Autodesk Inventor part; units mm, degrees
ref_plane "Arbeitsebene1" through (0, 1.75, 0) normal (0, 1, 0) x (-1, 0, 0)
ref_plane "YZ Plane" through (0, 0, 0) normal (1, 0, 0) x (0, 1, 0)
ref_plane "XY Plane" through (0, 0, 0) normal (0, 0, 1) x (1, 0, 0)
sketch "Skizze1" plane through (0, 0, 0) normal (0, 1, 0) x (-1, 0, 0)
  line L0 (0, 0) -> (1.5, 0)
  line L1 (1.5, 0) -> (1.5, -6.5)
  line L2 (1.5, -6.5) -> (2, -6.5)
  line L3 (2, -6.5) -> (2, -36.5)
  line L4 (0, 0) -> (0, -44)
  line L5 (2, -36.5) -> (1.5, -36.5)
  line L6 (1.5, -36.5) -> (1.5, -42.5)
  arc A0 (0, -44) -> (1.5, -42.5) centre (0, -42.5) ccw
  point P0 (0, -26.7554)
  dimension "d0" = 6.5
  dimension "d1" = 3
  dimension "d2" = 4
  dimension "d5" = 30
  dimension "d6" = 0.5
  dimension "d7" = 6
revolve "Umdrehung1" add sketch "Skizze1" angle 360 about axis through (0, 0, 0) along (0, 0, -1)
thread "Gewinde1"
ref_plane "Arbeitsebene1" through (0, 1.75, 0) normal (0, 1, 0) x (-1, 0, 0)
sketch "Skizze2" plane through (0, 1.75, 0) normal (0, 1, 0) x (-1, 0, 0)
  line L0 (-2, -36.5) -> (2, -36.5)
  point P0 (0, 0)
  point P1 (0, -40)
  dimension "d13" = 3.5
hole "Bohrung1" at (0, 1.75, -40) direction (0, -1, 0) diameter 2 end through all
properties part number "19_2"
Here's how the part is built. I have some questions about the finished solid (model axes, mm). A direction names the side the tool comes from. Coordinates: 2 decimals unless noted, no trailing zeros. Write each loop counter-clockwise with the first axis right and the second up, starting at its lowest first coordinate (ties: lowest second). Pieces come first, ordered by that corner, then holes. Notation, with made-up numbers: M 23.25,-30 L 81.25,-30 A27 ccw 81.25,8 Z; hole C -39.5,73 d11. An arc over 180 degrees is marked long. Answer as CSV lines item,"result". Start each with the question number.
Q1. Suppose I cut it at B-B, the plane y = 0. List the corners of the cut face in (x, z) for me.
Q2. I need wall thicknesses on probe 1 along Z at (x, y) = (0, 0.05); probe 2 along Z at (x, y) = (-1.7, 0.2); probe 3 along Z at (x, y) = (-0.65, 0.65). Which ranges of each line are inside material? Lowest first, please. Write a range as [from, to].
Q3. For faces 1 (the cylindrical face through (1.5, 0.07, -3.3)), 2 (the cylindrical face through (1.5, 0.07, -39.54)), which set-ups out of +Z, -Z, +X, -X, +Y, -Y let a thin tool reach every point of the face, with its end or its side?
Q4. Suppose I cut it at C-C, the plane z = -18.5. List the corners of the cut face in (x, y) for me, then the cut area to 3 significant figures.
Q5. Will these pins go through, and if not, where does the flat tip stop? pin 1 Ø1.5 at (x, z) = (1, -10) entering from +Y; pin 2 Ø1.2 at (x, y) = (-0.5, -0.5) entering from +Z; pin 3 Ø1.2 at (x, y) = (-1, 1) entering from -Z; pin 4 Ø1 at (y, z) = (1, -34) entering from +X.
Q6. Suppose I cut it at D-D, the plane z = -40. List the corners of the cut face in (x, y) for me.
Q7. Suppose I cut it at A-A, the plane x = 0. List the corners of the cut face in (y, z) for me, then the cut area to 3 significant figures.
Q8. If we mould it in two halves opening along Z, with no side actions, what happens to faces 3 (the flat face through (0, 0, 0)), 4 (the cylindrical face through (0, -2, -22)), 5 (the cylindrical face through (0.6, 0, -40.8))? For each: pulls with the +Z half, pulls with the -Z half, needs draft (parallel to the pull), parting line crosses it, or undercut.
Entries:
1,outline,"M -2,-36.5 L -1.5,-36.5 L -1.5,-42.5 A1.5 ccw 1.5,-42.5 L 1.5,-36.5 L 2,-36.5 L 2,-6.5 L 1.5,-6.5 L 1.5,0 L -1.5,0 L -1.5,-6.5 L -2,-6.5 Z; hole C 0,-40 d2"
2,probe 1,"z = [-44, -41], [-39, 0]"
2,probe 2,"z = [-36.5, -6.5]"
2,probe 3,"z = [-43.69, -40.76], [-39.24, 0]"
3,face 1,"+Z"
3,face 2,"-Z"
4,outline,"C 0,0 d4"
4,area,"12.6 mm²"
5,pin 1,"stops at y = 1.98"
5,pin 2,"stops at z = 0"
5,pin 3,"stops at z = -43.76"
5,pin 4,"stops at x = 1.94"
6,outline,"M -1,-1.12 L -1,1.12 A1.5 ccw Z; M 1,-1.12 A1.5 ccw 1,1.12 Z"
7,outline,"M -2,-36.5 L -1.5,-36.5 L -1.5,-39 L 1.5,-39 L 1.5,-36.5 L 2,-36.5 L 2,-6.5 L 1.5,-6.5 L 1.5,0 L -1.5,0 L -1.5,-6.5 L -2,-6.5 Z; M -1.5,-42.5 A1.5 ccw 1.5,-42.5 L 1.5,-41 L -1.5,-41 Z"
7,area,"155 mm²"
8,face 3,"pulls with the +Z half"
8,face 4,"needs draft"
8,face 5,"undercut"
